Autodesk Inventor part; units mm, degrees
ref_plane "YZ Plane" through (0, 0, 0) normal (1, 0, 0) x (0, 1, 0)
ref_plane "XZ Plane" through (0, 0, 0) normal (0, 1, 0) x (-1, 0, 0)
ref_plane "XY Plane" through (0, 0, 0) normal (0, 0, 1) x (1, 0, 0)
sketch "Skizze1" plane through (0, 0, 0) normal (0, 1, 0) x (-1, 0, 0)
  line L0 (-65, 30) -> (65, 30)
  line L1 (65, 30) -> (65, -30)
  line L2 (65, -30) -> (-65, -30)
  line L3 (-65, -30) -> (-65, 30)
  line L4 (0, -42) -> (0, 42)
  line L5 (-91, 0) -> (91, 0)
  point P0 (0, 0)
  dimension "d0" = 130
  dimension "d1" = 60
extrude "Extrusion1" add sketch "Skizze1" along normal blind 2
sketch "Skizze2" plane through (0, 2, 0) normal (0, 1, 0) x (1, 0, 0)
  line L0 (0, 42) -> (0, -42)
  line L1 (91, 0) -> (-91, 0)
  circle A0 centre (49.76, -24.13) radius 2.25
  line L2 (65, -30) -> (65, 30)
  circle A1 centre (51.03, 24.13) radius 2.25
  circle A2 centre (-31.52, 24.13) radius 2.25
  circle A3 centre (-25.17, -24.13) radius 2.25
  circle A4 centre (21.3223, -24.13) radius 2
  circle A5 centre (22.5923, 24.13) radius 2
  circle A6 centre (-59.9577, 24.13) radius 2
  circle A7 centre (-53.6077, -24.13) radius 2
  line L3 (-65, 30) -> (-65, -30)
  circle A8 centre (49.76, -24.13) radius 3.5
  circle A9 centre (-25.17, -24.13) radius 3.5
  circle A10 centre (51.03, 24.13) radius 3.5
  circle A11 centre (-31.52, 24.13) radius 3.5
  point P0 (0, 0)
  dimension "d4" = 4.5
  dimension "d5" = 24.13
  dimension "d6" = 15.24
  dimension "d7" = 4.5
  dimension "d8" = 24.13
  dimension "d9" = 13.97
  dimension "d10" = 4.5
  dimension "d11" = 24.13
  dimension "d12" = 82.55
  dimension "d13" = 4.5
  dimension "d14" = 24.13
  dimension "d15" = 74.93
  dimension "d16" = 4
  dimension "d17" = 4
  dimension "d18" = 4
  dimension "d19" = 82.55
  dimension "d20" = 4
  dimension "d21" = 74.93
  dimension "d22" = 24.13
  dimension "d23" = 24.13
  dimension "d24" = 11.3923
  dimension "d25" = 5.0423
  dimension "d26" = 24.13
  dimension "d27" = 24.13
  dimension "d41" = 7
  dimension "d42" = 7
  dimension "d43" = 7
  dimension "d44" = 7
extrude "Extrusion2" cut sketch "Skizze2" against normal up to surface (2 mm away) contours A0 | A1 | A2 | A3 | A4 | A5 | A6 | A7
sketch "Skizze3" plane through (0, 2, 0) normal (0, 1, 0) x (1, 0, 0)
  line L0 (-65, 30) -> (-65, -30)
  line L1 (-65, -17.5) -> (-30, -17.5)
  line L2 (-30, -17.5) -> (-30, 17.5)
  line L3 (-30, 17.5) -> (-65, 17.5)
  line L4 (-65, 17.5) -> (-65, -17.5)
  line L5 (91, 0) -> (-91, 0)
  line L6 (50, -17.5) -> (-20, -17.5)
  line L7 (-20, -17.5) -> (-20, 17.5)
  line L8 (-20, 17.5) -> (50, 17.5)
  line L9 (50, 17.5) -> (50, -17.5)
  line L10 (65, -30) -> (65, 30)
  point P0 (0, 0)
  dimension "d30" = 35
  dimension "d31" = 35
  dimension "d36" = 70
  dimension "d37" = 35
  dimension "d38" = 15
extrude "Extrusion3" cut sketch "Skizze3" against normal up to surface (2 mm away)
sketch "Skizze4" plane through (-65, 0, 30) normal (-1, 0, 0) x (0, 0, 1)
  line L0 (-12.5, 2) -> (-12.5, 0)
  line L1 (0, 0) -> (-12.5, 0)
  line L2 (-12.5, 0) -> (-12.5, 2)
  line L3 (-12.5, 2) -> (0, 2)
  line L4 (0, 2) -> (0, 0)
  line L5 (-60, 0) -> (-60, 2)
  line L6 (-47.5, 0) -> (-47.5, 2)
  line L7 (-60, 0) -> (-47.5, 0)
  line L8 (-47.5, 0) -> (-47.5, 2)
  line L9 (-47.5, 2) -> (-60, 2)
  line L10 (-60, 2) -> (-60, 0)
  point P0 (-30, 0)
extrude "Extrusion4" cut sketch "Skizze4" against normal blind 1
sketch "Skizze5" plane through (65, 0, 30) normal (1, 0, 0) x (0, 0, -1)
  line L0 (0, 0) -> (0, 2)
  line L1 (60, 0) -> (60, 2)
  line L2 (0, 2) -> (60, 2)
  line L3 (60, 2) -> (60, 0)
  line L4 (60, 0) -> (0, 0)
  line L5 (0, 0) -> (0, 2)
  point P0 (30, 0)
extrude "Extrusion5" cut sketch "Skizze5" against normal blind 8
extrude "Extrusion6" add sketch "Skizze2" along normal blind 4 contours A8 | A9 | A10 | A11
fillet "Rundung1" radius 4 4 edges at (-64, 1, -30) (-64, 1, -17.5) (-64, 1, 17.5) (-64, 1, 30)
fillet "Rundung2" radius 4 2 edges at (57, 1, 30) (57, 1, -30)
properties part number "_3D-Druck"
Can you work these out from the model? Positions are in its coordinate system, mm. A direction names the side the tool comes from. Round coordinates to 2 decimals unless told otherwise and drop trailing zeros. Loops run counter-clockwise (first coordinate to the right, second up) from the corner with the lowest first, then second, coordinate; pieces in that order, holes last. Notation, with made-up numbers: (63.5, 82.25) -> (105.5, 82.25) arc R30 ccw to (105.5, 113.25) -> close; hole circle Ø9 at (88.5, -29.75). An arc over 180 degrees is marked (long way). One line per item, written item: value. Start each with the question number.
1. If we section it at B-B, the plane x = -31.52: Write out the boundary of the cut face in (y, z).
2. If I drill on probe 1 along X at (y, z) = (1.35, 24.13); probe 2 along X at (y, z) = (4.6, 24.13); probe 3 along Z at (x, y) = (-4, 0.5), over which ranges is the centre line in solid material (lowest first)?
3. If we section it at C-C, the plane z = -24.13: Write out the boundary of the cut face in (x, y).
4. If we mould it in two halves opening along X, with no side actions, what happens to faces 1 (the cylindrical face through (-30.31, 2.958, -22.233)), 2 (the cylindrical face through (-62.859, 0.986, 18.703)), 3 (the cylindrical face through (55.797, 1.014, 28.859))? For each: pulls with the +X half, pulls with the -X half, needs draft (parallel to the pull), parting line crosses it, or undercut.
5. For faces 4 (the cylindrical face through (-29.64, 3.97, -21.18)), 5 (the cylindrical face through (51.906, 2.958, 24.806)), which set-ups out of +Z, -Z, +X, -X, +Y, -Y let a thin tool reach every point of the face, with its end or its side?
6. If we section it at D-D, the plane x = 10.5: Write out the boundary of the cut face in (y, z), then the cut area to 3 significant figures.
7. If we section it at A-A, the plane y = 3.75: Write out the boundary of the cut face in (x, z).
8. For pin 1 (2.5 mm diameter, centred on x = 49.76, z = 24.13, fed in from -Y); pin 2 (18 mm diameter, centred on x = -27.5, z = -6, fed in from +Y); pin 3 (1.6 mm diameter, centred on y = 1.5, z = -4, fed in from -X), each with a flat end and sliding along its axis, tell me the tip position at first contact or that it passes through.
Calculated:
1. outline: (0, -30) -> (2, -30) -> (2, -27.63) -> (6, -27.63) -> (6, -26.38) -> (0, -26.38) -> close; (0, -21.88) -> (6, -21.88) -> (6, -20.63) -> (2, -20.63) -> (2, -17.5) -> (0, -17.5) -> close; (0, 17.5) -> (2, 17.5) -> (2, 30) -> (0, 30) -> close
2. probe 1: x = -64 to -55.61, -51.61 to -27.42, -22.92 to 19.32, 23.32 to 47.51, 52.01 to 57
2. probe 2: x = -28.67 to -27.42, -22.92 to -21.67, 46.26 to 47.51, 52.01 to 53.26
2. probe 3: z = -30 to -17.5, 17.5 to 30
3. outline: (-64, 0) -> (-61.96, 0) -> (-61.96, 2) -> (-64, 2) -> close; (-57.96, 0) -> (-33.77, 0) -> (-33.77, 6) -> (-35.02, 6) -> (-35.02, 2) -> (-57.96, 2) -> close; (-29.27, 0) -> (20.59, 0) -> (20.59, 2) -> (-28.02, 2) -> (-28.02, 6) -> (-29.27, 6) -> close; (24.59, 0) -> (48.78, 0) -> (48.78, 6) -> (47.53, 6) -> (47.53, 2) -> (24.59, 2) -> close; (53.28, 0) -> (57, 0) -> (57, 2) -> (54.53, 2) -> (54.53, 6) -> (53.28, 6) -> close
4. face 1: undercut
4. face 2: pulls with the -X half
4. face 3: pulls with the +X half
5. face 4: +Y
5. face 5: +Y, -Y
6. outline: (0, -30) -> (2, -30) -> (2, -17.5) -> (0, -17.5) -> close; (0, 17.5) -> (2, 17.5) -> (2, 30) -> (0, 30) -> close
6. area: 50.0 mm²
7. outline: circle Ø7 at (-31.52, -24.13); circle Ø7 at (-25.17, 24.13); circle Ø7 at (49.76, 24.13); circle Ø7 at (51.03, -24.13); hole circle Ø4.5 at (-31.52, -24.13); hole circle Ø4.5 at (-25.17, 24.13); hole circle Ø4.5 at (49.76, 24.13); hole circle Ø4.5 at (51.03, -24.13)
8. pin 1: passes through
8. pin 2: stops at y = 2
8. pin 3: stops at x = -30
